from build123d import *

# Parameters (mm, degrees)
BOSS_EXTRUDE1_DEPTH = 90
SHELL1_T            = -3
FILLET1_R           = 2
SKETCH3_R           = 1.35
CUT_EXTRUDE1_DEPTH  = 3


with BuildPart() as part:
    # Sketch2 → Boss-Extrude1 (new body)
    with BuildSketch(Plane(origin=(0, 0, 0), x_dir=(1, 0, 0), z_dir=(0, 1, 0))):
        with BuildLine():
            Line((-145, 100), (145, 100))
            ThreePointArc((145, 100), (148.535533906, 98.535533906), (150, 95))
            Line((150, 95), (150, -95))
            ThreePointArc((150, -95), (148.535533906, -98.535533906), (145, -100))
            Line((145, -100), (-145, -100))
            ThreePointArc((-145, -100), (-148.535533906, -98.535533906), (-150, -95))
            Line((-150, -95), (-150, 95))
            ThreePointArc((-150, 95), (-148.535533906, 98.535533906), (-145, 100))
        make_face()
    extrude(amount=BOSS_EXTRUDE1_DEPTH)

    # Shell1
    shell1_openings = [part.faces().sort_by_distance(p)[0] for p in [
        (0, 90, 0),
    ]]
    offset(amount=SHELL1_T, openings=shell1_openings, kind=Kind.INTERSECTION)

    # Fillet1
    fillet1_edges = [part.edges().sort_by_distance(p)[0] for p in [
        (150, 0, 0),
        (148.535533906, 0, 98.535533906),
        (0, 0, 100),
        (-148.535533906, 0, 98.535533906),
        (-150, 0, 0),
        (-148.535533906, 0, -98.535533906),
        (0, 0, -100),
        (148.535533906, 0, -98.535533906),
    ]]
    fillet(fillet1_edges, radius=FILLET1_R)

    # Sketch3 → Cut-Extrude1 (cut)
    with BuildSketch(Plane(origin=(0, 3, 0), x_dir=(1, 0, 0), z_dir=(0, 1, 0))):
        with Locations(Location((-99.315591438, -29, 0), (0, 0, 270))):
            Circle(SKETCH3_R)
        with Locations(Location((-50.315591438, -29, 0), (0, 0, 270))):
            Circle(SKETCH3_R)
        with Locations(Location((-50.315591438, 29, 0), (0, 0, 270))):
            Circle(SKETCH3_R)
        with Locations(Location((-99.315591438, 29, 0), (0, 0, 270))):
            Circle(SKETCH3_R)
        with Locations(Location((87.050591438, -12.235, 0), (0, 0, 270))):
            Circle(SKETCH3_R)
        with Locations(Location((87.050591438, 12.235, 0), (0, 0, 270))):
            Circle(SKETCH3_R)
        with Locations(Location((62.580591438, 12.235, 0), (0, 0, 270))):
            Circle(SKETCH3_R)
        with Locations(Location((62.580591438, -12.235, 0), (0, 0, 270))):
            Circle(SKETCH3_R)
    extrude(amount=-CUT_EXTRUDE1_DEPTH, mode=Mode.SUBTRACT)


solid = part.part
Design review of the part built by this model. Coordinates are the model's own, in mm. A direction names the side the tool comes from. Coordinates: 2 decimals unless noted, no trailing zeros. Loops run counter-clockwise (first coordinate to the right, second up) from the corner with the lowest first, then second, coordinate; pieces in that order, holes last. Notation, with made-up numbers: (79.5, 89.5) -> (103.5, 89.5) arc R21 ccw to (103.5, 102.5) -> close; hole circle Ø7 at (48.5, 14.5). An arc over 180 degrees is marked (long way). Use a Markdown table: item, result. Add a question column.
Item 1: We need section B-B, the plane z = 83. Write out the cut boundary in (x, y).
Item 2: The part is to be moulded in two halves that separate along Z. For faces 3 (the flat face through (-2, 46, -97)), 4 (the flat face through (-147, 46, 1)), 5 (the flat face through (2, 45, 100)), 6 (the flat face through (-150, 45, 1)), say which applies: +Z half, -Z half, draft (parallel to the pull), parting line (faces both ways), or undercut.
Item 3: Wall thickness on L1, parallel to X at y = 60, z = 29; L2, parallel to Z at x = -70, y = 71.5; L3, parallel to X at y = 1.6, z = -29: over which ranges is each line inside the solid? List them lowest first. Write a range as from..to.
Item 4: Clearance check with flat-ended pins moving along their axes: P1, Ø1.6, axis at x = -50.32, z = 29, coming from the +Y side; P2, Ø3, axis at x = 4, z = -0.5, coming from the +Y side. State where each tip first meets the part, or that it passes through.
Item 5: We need section C-C, the plane x = -60. Write out the cut boundary in (y, z), and give its area (3 significant figures).
Item 6: We need section A-A, the plane y = 42. Write out the cut boundary in (x, z).
Item 7: Machinability: for faces 1 (the flat face through (147, 46, -1)), 2 (the flat face through (2, 0, -1)), which of the approach directions +Z, -Z, +X, -X, +Y, -Y give a long, thin tool a straight path to every point of the face, cutting with its end or side? Answer none if there is none.
Numbers:
| question | item | result |
|---|---|---|
| 1 | outline | (-150, 2) arc R2 ccw to (-148, 0) -> (148, 0) arc R2 ccw to (150, 2) -> (150, 90) -> (147, 90) -> (147, 3) -> (-147, 3) -> (-147, 90) -> (-150, 90) -> close |
| 2 | face 3 | undercut |
| 2 | face 4 | undercut |
| 2 | face 5 | +Z half |
| 2 | face 6 | draft |
| 3 | L1 | x = -150..-147, 147..150 |
| 3 | L2 | z = -100..-97, 97..100 |
| 3 | L3 | x = -149.96..-100.67, -97.97..-51.67, -48.97..149.96 |
| 4 | P1 | passes through |
| 4 | P2 | stops at y = 3 |
| 5 | outline | (0, -98) arc R2 ccw to (2, -100) -> (90, -100) -> (90, -97) -> (3, -97) -> (3, 97) -> (90, 97) -> (90, 100) -> (2, 100) arc R2 ccw to (0, 98) -> close |
| 5 | area | 1,120 mm^2 |
| 6 | outline | (-150, -95) arc R5 ccw to (-145, -100) -> (145, -100) arc R5 ccw to (150, -95) -> (150, 95) arc R5 ccw to (145, 100) -> (-145, 100) arc R5 ccw to (-150, 95) -> close; hole (-147, -95) arc R2 ccw to (-145, -97) -> (145, -97) arc R2 ccw to (147, -95) -> (147, 95) arc R2 ccw to (145, 97) -> (-145, 97) arc R2 ccw to (-147, 95) -> close |
| 7 | face 1 | +Y |
| 7 | face 2 | +Z, -Z, +X, -X, -Y |
